Source: three-view drawing plus pictorial views. Frame: mm from the lowest corner of the part. Give positions to 0.01 mm unless a question says otherwise; leave off trailing zeros. Loops run counter-clockwise (first coordinate to the right, second up) from the corner with the lowest first, then second, coordinate; pieces in that order, holes last.
1. Section A-A, the plane z = 10. Output: boundary loops of the cut face in (x, y), then the cut area to 4 significant figures.
2. First-contact query: P1, Ø2, axis at x = 32.5, z = 25, coming from the -Y side; P2, Ø4.5, axis at x = 10, z = 10, coming from the -Y side. Flat tips, straight axial feed; report the tip coordinate or a pass-through.
3. Material intervals for line 1 along Z through (x, y) = (130, 0.65), sorted ascending.
4. Section B-B, the plane x = 130. Output: boundary loops of the cut face in (y, z).
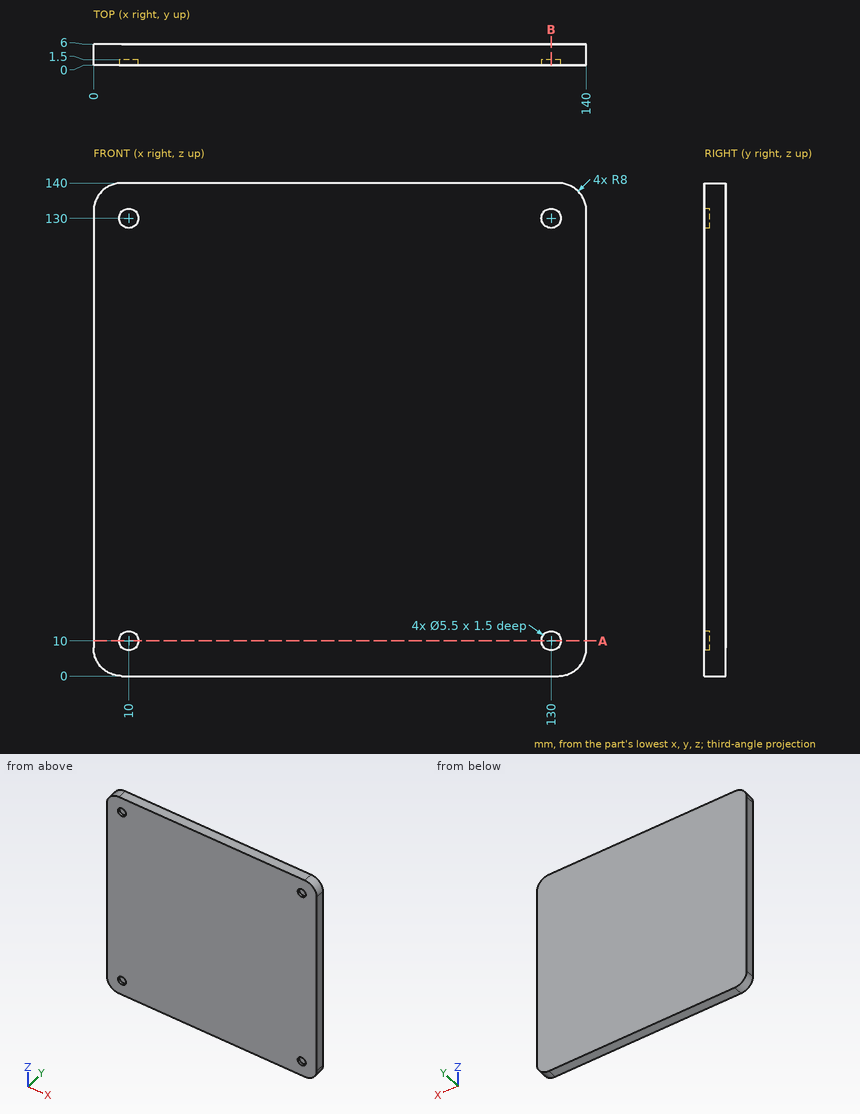
Answers below:
1. outline: (0, 0) - (7.25, 0) - (7.25, 1.5) - (12.75, 1.5) - (12.75, 0) - (127.25, 0) - (127.25, 1.5) - (132.75, 1.5) - (132.75, 0) - (140, 0) - (140, 6) - (0, 6) - close
1. area: 823.5 mm2
2. P1: stops at y = 0
2. P2: stops at y = 1.5
3. line 1: z = 0 to 7.25, 12.75 to 127.25, 132.75 to 140
4. outline: (0, 0) - (6, 0) - (6, 140) - (0, 140) - (0, 132.75) - (1.5, 132.75) - (1.5, 127.25) - (0, 127.25) - (0, 12.75) - (1.5, 12.75) - (1.5, 7.25) - (0, 7.25) - close
